from build123d import *

# Parameters (mm, degrees)
SKETCH1_W                      = 54
SKETCH1_H                      = 23.8
BASE_FLANGE1_DEPTH             = 1
EDGE_FLANGE1_STRIP_W           = 5
EDGE_FLANGE1_STRIP_H           = 1
EDGE_FLANGE1_STRIP_CUT_DEPTH   = 54
EDGE_FLANGE1_STRIP_2_W         = 5
EDGE_FLANGE1_STRIP_2_H         = 1
EDGE_FLANGE1_STRIP_CUT_2_DEPTH = 54
EDGE_FLANGE1_DEPTH             = 54
EDGE_FLANGE1_BEND_DEPTH        = 54
EDGE_FLANGE2_STRIP_W           = 5
EDGE_FLANGE2_STRIP_H           = 1
EDGE_FLANGE2_STRIP_CUT_DEPTH   = 20.8
EDGE_FLANGE2_DEPTH             = 20.8
CUT_EXTRUDE1_START             = -1.5
CUT_EXTRUDE1_DEPTH             = 1.5
CUT_EXTRUDE2_START             = -1.5
CUT_EXTRUDE2_DEPTH             = 1.5
EDGE_FLANGE3_STRIP_W           = 5
EDGE_FLANGE3_STRIP_H           = 1
EDGE_FLANGE3_STRIP_CUT_DEPTH   = 54
EDGE_FLANGE3_STRIP_2_W         = 5
EDGE_FLANGE3_STRIP_2_H         = 1
EDGE_FLANGE3_STRIP_CUT_2_DEPTH = 54
EDGE_FLANGE3_DEPTH             = 54
EDGE_FLANGE3_BEND_DEPTH        = 54
BREAK_CORNER1_START            = -28.5
BREAK_CORNER1_DEPTH            = 1
CUT_EXTRUDE3_DEPTH             = 10
CUT_EXTRUDE4_DEPTH             = 2
CUT_EXTRUDE4_DEPTH_BACK        = 2
BREAK_CORNER2_START            = -28.5
BREAK_CORNER2_DEPTH            = 1
CUT_EXTRUDE5_DEPTH             = 1
SKETCH26_W                     = 2.9
SKETCH26_H                     = 5.9
CUT_EXTRUDE6_DEPTH             = 1
SKETCH27_R                     = 1.6
CUT_EXTRUDE7_DEPTH             = 1
MOVE_FACE1_BY                  = 0.15
MOVE_FACE1_2_BY                = 0.15
CHAMFER1_SIZE                  = 1
CHAMFER2_SIZE                  = 1


# Read off the part's stored shape, not the designer's step: Break-Corner1, Break-Corner2
# Sheet-metal steps are written as plain solids
# Some blends are built 0.0001 mm under size
with BuildPart() as part:
    # Sketch1 → Base-Flange1 (new body)
    with BuildSketch(Plane(origin=(0, 0, 0), x_dir=(1, 0, 0), z_dir=(0, 1, 0))):
        Rectangle(SKETCH1_W, SKETCH1_H)
    extrude(amount=-BASE_FLANGE1_DEPTH)

    # Edge-Flange1 strip (across the edge) → Edge-Flange1 strip cut (cut)
    with BuildSketch(Plane(origin=(27, -1, 11.9), x_dir=(0, 0, -1), z_dir=(-1, 0, 0))):
        with Locations((-1, -0.5)):
            Rectangle(EDGE_FLANGE1_STRIP_W, EDGE_FLANGE1_STRIP_H)
    extrude(amount=EDGE_FLANGE1_STRIP_CUT_DEPTH, mode=Mode.SUBTRACT)

    # Edge-Flange1 strip 2 (across the edge) → Edge-Flange1 strip cut 2 (cut)
    with BuildSketch(Plane(origin=(-27, -1, -11.9), x_dir=(0, 0, 1), z_dir=(1, 0, 0))):
        with Locations((-1, -0.5)):
            Rectangle(EDGE_FLANGE1_STRIP_2_W, EDGE_FLANGE1_STRIP_2_H)
    extrude(amount=EDGE_FLANGE1_STRIP_CUT_2_DEPTH, mode=Mode.SUBTRACT)

    # Edge-Flange1 section (across the edge) → Edge-Flange1 (add)
    with BuildSketch(Plane(origin=(27, -1, 11.9), x_dir=(0, 0, -1), z_dir=(-1, 0, 0))):
        with BuildLine():
            Line((0, 0.5), (0, 27.5))
            Line((0, 27.5), (1, 27.5))
            Line((1, 27.5), (1, 0.5))
            ThreePointArc((1, 0.5), (1.146446609, 0.146446609), (1.5, 0))
            Line((1.5, 0), (1.5, -1))
            ThreePointArc((1.5, -1), (0.439339828, -0.560660172), (0, 0.5))
        make_face()
    extrude(amount=EDGE_FLANGE1_DEPTH)

    # Edge-Flange1 section 2 (across the edge) → Edge-Flange1 bend (add)
    with BuildSketch(Plane(origin=(-27, -1, -11.9), x_dir=(0, 0, 1), z_dir=(1, 0, 0))):
        with BuildLine():
            Line((0, 0.5), (0, 27.5))
            Line((0, 27.5), (1, 27.5))
            Line((1, 27.5), (1, 0.5))
            ThreePointArc((1, 0.5), (1.146446609, 0.146446609), (1.5, 0))
            Line((1.5, 0), (1.5, -1))
            ThreePointArc((1.5, -1), (0.439339828, -0.560660172), (0, 0.5))
        make_face()
    extrude(amount=EDGE_FLANGE1_BEND_DEPTH)

    # Edge-Flange2 strip (across the edge) → Edge-Flange2 strip cut (cut)
    with BuildSketch(Plane(origin=(27, -1, -10.4), x_dir=(-1, 0, 0), z_dir=(0, 0, 1))):
        with Locations((-1, -0.5)):
            Rectangle(EDGE_FLANGE2_STRIP_W, EDGE_FLANGE2_STRIP_H)
    extrude(amount=EDGE_FLANGE2_STRIP_CUT_DEPTH, mode=Mode.SUBTRACT)

    # Edge-Flange2 section (across the edge) → Edge-Flange2 (add)
    with BuildSketch(Plane(origin=(27, -1, -10.4), x_dir=(-1, 0, 0), z_dir=(0, 0, 1))):
        with BuildLine():
            Line((0, 0.5), (0, 1.5))
            Line((0, 1.5), (1, 1.5))
            Line((1, 1.5), (1, 0.5))
            ThreePointArc((1, 0.5), (1.146446609, 0.146446609), (1.5, 0))
            Line((1.5, 0), (1.5, -1))
            ThreePointArc((1.5, -1), (0.439339828, -0.560660172), (0, 0.5))
        make_face()
    extrude(amount=EDGE_FLANGE2_DEPTH)

    # Sketch15 → Cut-Extrude1 (cut)
    with BuildSketch(Plane(origin=(0, 0, -11.9), x_dir=(-1, 0, 0), z_dir=(0, 0, -1)).offset(CUT_EXTRUDE1_START)):
        Polygon((-27, -2.5), (-25.5, -2.5), (-25.5, 0), (-28.102393481, 0), (-28.102393481, -2.5), align=None)
    extrude(amount=CUT_EXTRUDE1_DEPTH, mode=Mode.SUBTRACT)

    # Sketch16 → Cut-Extrude2 (cut)
    with BuildSketch(Plane.XY.offset(11.9).offset(CUT_EXTRUDE2_START)):
        Polygon((25.5, -2.5), (25.5, 0), (28.102393481, 0), (28.102393481, -2.5), (27, -2.5), align=None)
    extrude(amount=CUT_EXTRUDE2_DEPTH, mode=Mode.SUBTRACT)

    # Edge-Flange3 strip (across the edge) → Edge-Flange3 strip cut (cut)
    with BuildSketch(Plane(origin=(-27, -28.5, 11.9), x_dir=(0, 1, 0), z_dir=(1, 0, 0))):
        with Locations((-1, -0.5)):
            Rectangle(EDGE_FLANGE3_STRIP_W, EDGE_FLANGE3_STRIP_H)
    extrude(amount=EDGE_FLANGE3_STRIP_CUT_DEPTH, mode=Mode.SUBTRACT)

    # Edge-Flange3 strip 2 (across the edge) → Edge-Flange3 strip cut 2 (cut)
    with BuildSketch(Plane(origin=(27, -28.5, -11.9), x_dir=(0, 1, 0), z_dir=(-1, 0, 0))):
        with Locations((-1, -0.5)):
            Rectangle(EDGE_FLANGE3_STRIP_2_W, EDGE_FLANGE3_STRIP_2_H)
    extrude(amount=EDGE_FLANGE3_STRIP_CUT_2_DEPTH, mode=Mode.SUBTRACT)

    # Edge-Flange3 section (across the edge) → Edge-Flange3 (add)
    with BuildSketch(Plane(origin=(-27, -28.5, 11.9), x_dir=(0, 1, 0), z_dir=(1, 0, 0))):
        with BuildLine():
            Line((0, 0.5), (0, 8))
            Line((0, 8), (1, 8))
            Line((1, 8), (1, 0.5))
            ThreePointArc((1, 0.5), (1.146446609, 0.146446609), (1.5, 0))
            Line((1.5, 0), (1.5, -1))
            ThreePointArc((1.5, -1), (0.439339828, -0.560660172), (0, 0.5))
        make_face()
    extrude(amount=EDGE_FLANGE3_DEPTH)

    # Edge-Flange3 section 2 (across the edge) → Edge-Flange3 bend (add)
    with BuildSketch(Plane(origin=(27, -28.5, -11.9), x_dir=(0, 1, 0), z_dir=(-1, 0, 0))):
        with BuildLine():
            Line((0, 0.5), (0, 8))
            Line((0, 8), (1, 8))
            Line((1, 8), (1, 0.5))
            ThreePointArc((1, 0.5), (1.146446609, 0.146446609), (1.5, 0))
            Line((1.5, 0), (1.5, -1))
            ThreePointArc((1.5, -1), (0.439339828, -0.560660172), (0, 0.5))
        make_face()
    extrude(amount=EDGE_FLANGE3_BEND_DEPTH)

    # Break-Corner1 outline → Break-Corner1 (cut)
    with BuildSketch(Plane(origin=(0, 0, 0), x_dir=(1, 0, 0), z_dir=(0, 1, 0)).offset(BREAK_CORNER1_START)):
        with BuildLine():
            Line((-27, -19.9), (-24.5, -19.9))
            ThreePointArc((-24.5, -19.9), (-26.267766953, -19.167766953), (-27, -17.4))
            Line((-27, -17.4), (-27, -19.9))
        make_face()
        with BuildLine():
            ThreePointArc((27, -17.4), (26.267766953, -19.167766953), (24.5, -19.9))
            Line((24.5, -19.9), (27, -19.9))
            Line((27, -19.9), (27, -17.4))
        make_face()
        with BuildLine():
            Line((27, 19.9), (24.5, 19.9))
            ThreePointArc((24.5, 19.9), (26.267766953, 19.167766953), (27, 17.4))
            Line((27, 17.4), (27, 19.9))
        make_face()
        with BuildLine():
            ThreePointArc((-27, 17.4), (-26.267766953, 19.167766953), (-24.5, 19.9))
            Line((-24.5, 19.9), (-27, 19.9))
            Line((-27, 19.9), (-27, 17.4))
        make_face()
    extrude(amount=BREAK_CORNER1_DEPTH, mode=Mode.SUBTRACT)

    # Sketch23 → Cut-Extrude3 (cut)
    with BuildSketch(Plane(origin=(0, -27.5, 0), x_dir=(1, 0, 0), z_dir=(0, 1, 0))):
        with BuildLine():
            Line((13.35, 17.9), (16.95, 17.9))
            ThreePointArc((16.95, 17.9), (18.5, 16.35), (16.95, 14.8))
            Line((16.95, 14.8), (13.35, 14.8))
            ThreePointArc((13.35, 14.8), (11.8, 16.35), (13.35, 17.9))
        make_face()
        with BuildLine():
            Line((-13.35, 14.8), (-16.95, 14.8))
            ThreePointArc((-16.95, 14.8), (-18.5, 16.35), (-16.95, 17.9))
            Line((-16.95, 17.9), (-13.35, 17.9))
            ThreePointArc((-13.35, 17.9), (-11.8, 16.35), (-13.35, 14.8))
        make_face()
        with BuildLine():
            Line((13.35, -17.9), (16.95, -17.9))
            ThreePointArc((16.95, -17.9), (18.5, -16.35), (16.95, -14.8))
            Line((16.95, -14.8), (13.35, -14.8))
            ThreePointArc((13.35, -14.8), (11.8, -16.35), (13.35, -17.9))
        make_face()
        with BuildLine():
            Line((-13.35, -14.8), (-16.95, -14.8))
            ThreePointArc((-16.95, -14.8), (-18.5, -16.35), (-16.95, -17.9))
            Line((-16.95, -17.9), (-13.35, -17.9))
            ThreePointArc((-13.35, -17.9), (-11.8, -16.35), (-13.35, -14.8))
        make_face()
    extrude(amount=-CUT_EXTRUDE3_DEPTH, mode=Mode.SUBTRACT)

    # Sketch24 → Cut-Extrude4 (cut, two sides: drawn at the far end of the back side and taken through both)
    with BuildSketch(Plane(origin=(0, 0, -11.9), x_dir=(-1, 0, 0), z_dir=(0, 0, -1)).offset(-CUT_EXTRUDE4_DEPTH_BACK)):
        with BuildLine():
            Line((27, -28.5), (20.7, -28.5))
            Line((20.7, -28.5), (20.7, -26))
            ThreePointArc((20.7, -26), (21.432233047, -24.232233047), (23.2, -23.5))
            Line((23.2, -23.5), (27, -23.5))
            Line((27, -23.5), (27, -28.5))
        make_face()
    extrude(amount=CUT_EXTRUDE4_DEPTH + CUT_EXTRUDE4_DEPTH_BACK, mode=Mode.SUBTRACT)

    # Break-Corner2 outline → Break-Corner2 (add)
    with BuildSketch(Plane(origin=(0, 0, 0), x_dir=(1, 0, 0), z_dir=(0, 1, 0)).offset(BREAK_CORNER2_START)):
        with BuildLine():
            Line((-20.7, 13.9), (-22.2, 13.9))
            ThreePointArc((-22.2, 13.9), (-21.139339828, 13.460660172), (-20.7, 12.4))
            Line((-20.7, 12.4), (-20.7, 13.9))
        make_face()
    extrude(amount=BREAK_CORNER2_DEPTH)

    # Sketch25 → Cut-Extrude5 (cut)
    with BuildSketch(Plane.XY.offset(-10.9)):
        Polygon((27, -10.2), (23.6, -10.2), (23.6, -11.7), (25.3, -11.7), (25.3, -17.6), (23.6, -17.6), (23.6, -19.1), (27, -19.1), align=None)
    extrude(amount=-CUT_EXTRUDE5_DEPTH, mode=Mode.SUBTRACT)

    # Sketch26 → Cut-Extrude6 (cut)
    with BuildSketch(Plane.XY.offset(11.9)):
        with Locations((25.55, -13.95)):
            Rectangle(SKETCH26_W, SKETCH26_H)
    extrude(amount=-CUT_EXTRUDE6_DEPTH, mode=Mode.SUBTRACT)

    # Sketch27 → Cut-Extrude7 (cut)
    with BuildSketch(Plane(origin=(0, 0, 0), x_dir=(1, 0, 0), z_dir=(0, 1, 0))):
        with Locations(Location((-16.6, -7.3, 0), (0, 0, 270))):
            Circle(SKETCH27_R)
        with Locations(Location((3.4, 7.8, 0), (0, 0, 270))):
            Circle(SKETCH27_R)
    extrude(amount=-CUT_EXTRUDE7_DEPTH, mode=Mode.SUBTRACT)

    # Move Face1: a curved face moved inward by 0.15
    add(Solid.thicken(part.faces().sort_by_distance((3.4, -0.5, -9.4))[0], -MOVE_FACE1_BY), mode=Mode.SUBTRACT)

    # Move Face1 2: a curved face moved inward by 0.15
    add(Solid.thicken(part.faces().sort_by_distance((-16.6, -0.5, 5.7))[0], -MOVE_FACE1_2_BY), mode=Mode.SUBTRACT)

    # Chamfer1
    chamfer1_edges = [part.edges().sort_by_distance(p)[0] for p in [
        (-16.6, 0, 5.55),
    ]]
    chamfer(chamfer1_edges, length=CHAMFER1_SIZE - 0.0001)  # a hair under: the kernel refuses the full size

    # Chamfer2
    # the kernel refuses this chamfer: 1 mm, written as the material it takes off along each edge
    with BuildSketch(Plane(origin=(3.4, 0, -7.8), x_dir=(0, 0, 1), z_dir=(-1, 0, 0))) as chamfer2_piece_1:
        Polygon((1.75 + CHAMFER2_SIZE, 0), (1.75, -CHAMFER2_SIZE), (1.75, 0), align=None)
    revolve(axis=Axis((3.4, 0, -7.8), (0, 1, 0)), mode=Mode.SUBTRACT)


solid = part.part
Can you work these out from the model? Positions are in its coordinate system, mm. A direction names the side the tool comes from. Give positions to 0.01 mm unless a question says otherwise; leave off trailing zeros. Write each loop counter-clockwise with the first axis right and the second up, starting at its lowest first coordinate (ties: lowest second). Pieces come first, ordered by that corner, then holes. Notation, with made-up numbers: M 53,52 L 98,52 A30 cw 98,82 Z; hole C 62.25,-28 d10. An arc over 180 degrees is marked long. Answer in a Markdown table with one row per item. Add a question column.
Item 1: For pin 1 Ø1.5 at (y, z) = (-8.5, 14) entering from -X; pin 2 Ø6 at (x, z) = (-6, -16) entering from +Y; pin 3 Ø1.2 at (y, z) = (-26.5, -12) entering from -X; pin 4 Ø0.8 at (x, z) = (26.5, 11.5) entering from +Y, each with a flat end and sliding along its axis, tell me the tip position at first contact or that it passes through.
Item 2: Imagine slicing it at C-C, the plane z = -16.35. Write out the boundary of the cut face in (x, y), plus the area to 3 significant figures.
Item 3: Imagine slicing it at D-D, the plane x = -10. Write out the boundary of the cut face in (y, z), plus the area to 3 significant figures.
Item 4: Please list where these lines run through material, in increasing order: L1, parallel to Z at x = -6, y = -9.5; L2, parallel to Y at x = -18.5, z = -3; L3, parallel to Y at x = -14, z = -14.5.
Item 5: We'd pull the mould along X, two halves only. Please class faces 1 (the cylindrical face through (-21.413, -24.252, -11.393)), 2 (the flat face through (-1, -1, 0)), 3 (the cylindrical face through (-18.5, -28, 16.3)): released by +X, released by -X, zero draft, split by the parting line, or undercut.
Item 6: Imagine slicing it at A-A, the plane y = -4. Write out the boundary of the cut face in (x, z), plus the area to 3 significant figures.
Item 7: On a 3-axis mill with a long thin cutter (end or side, diameter ignored), from which of +Z, -Z, +X, -X, +Y, -Y can I reach the whole of each face in a straight line? I mean faces 4 (the cylindrical face through (-11.8, -28, 16.4)), 5 (the flat face through (26, -1, 10.4)), 6 (the flat face through (-20.7, -27.3, -11.6)). Say none if no direction works.
Evaluation:
| question | item | result |
|---|---|---|
| 1 | pin 1 | passes through |
| 1 | pin 2 | stops at y = -27.5 |
| 1 | pin 3 | stops at x = -20.7 |
| 1 | pin 4 | stops at y = -2.5 |
| 2 | outline | M -27,-28.5 L -18.5,-28.5 L -18.5,-27.5 L -27,-27.5 Z; M -11.8,-28.5 L 11.8,-28.5 L 11.8,-27.5 L -11.8,-27.5 Z; M 18.5,-28.5 L 27,-28.5 L 27,-27.5 L 18.5,-27.5 Z |
| 2 | area | 40.6 mm² |
| 3 | outline | M -28.5,-19.9 L -27.5,-19.9 L -27.5,-12.4 A0.5 cw -27,-11.9 L -1.5,-11.9 A1.5 ccw 0,-10.4 L 0,10.4 A1.5 ccw -1.5,11.9 L -27,11.9 A0.5 cw -27.5,12.4 L -27.5,19.9 L -28.5,19.9 L -28.5,12.4 A1.5 ccw -27,10.9 L -1.5,10.9 A0.5 cw -1,10.4 L -1,-10.4 A0.5 cw -1.5,-10.9 L -27,-10.9 A1.5 ccw -28.5,-12.4 Z |
| 3 | area | 93.1 mm² |
| 4 | L1 | z = -11.9 to -10.9, 10.9 to 11.9 |
| 4 | L2 | y = -1 to 0 |
| 4 | L3 | y = -28.5 to -27.5 |
| 5 | face 1 | released by -X |
| 5 | face 2 | zero draft |
| 5 | face 3 | undercut |
| 6 | outline | M -27,-11.9 L 27,-11.9 L 27,-10.9 L -27,-10.9 Z; M -27,10.9 L 27,10.9 L 27,11.9 L -27,11.9 Z |
| 6 | area | 108 mm² |
| 7 | face 4 | +Y, -Y |
| 7 | face 5 | +Z, +X, +Y, -Y |
| 7 | face 6 | -X, -Y |
